Check sheet for the modelled part. Datum: model origin and axes. Units: mm. Give positions to 0.01 mm unless a question says otherwise; leave off trailing zeros. Answer in a Markdown table with one row per item.
from build123d import *

# Parameters (mm, degrees)
EXTRUDE_4_DEPTH = 155


with BuildPart() as part:
    # 草图1 → 凸台-拉伸4 (new body)
    with BuildSketch(Plane.XY):
        with BuildLine():
            Line((1.654438254, 0.021809694), (0.999524111, 15.021809694))
            ThreePointArc((0.999524111, 15.021809694), (0.489092557, 15.499881014), (0, 15))
            Line((0, 15), (0, 0))
            Line((0, 0), (0.5, 0))
            Line((0.5, 0), (0.5, 15))
            Line((0.5, 15), (1.154914144, 0))
            ThreePointArc((1.154914144, 0), (1.654438254, -0.478190306), (2.153962365, 0))
            Line((2.153962365, 0), (2.808876509, 15))
            Line((2.808876509, 15), (3.463790652, 0))
            ThreePointArc((3.463790652, 0), (3.963314763, -0.478190306), (4.462838874, 0))
            Line((4.462838874, 0), (5.117753018, 15))
            Line((5.117753018, 15), (5.772667161, 0))
            ThreePointArc((5.772667161, 0), (6.272191272, -0.478190306), (6.771715383, 0))
            Line((6.771715383, 0), (7.426629527, 15))
            Line((7.426629527, 15), (8.08154367, 0))
            ThreePointArc((8.08154367, 0), (8.581067781, -0.478190306), (9.080591892, 0))
            Line((9.080591892, 0), (9.735506035, 15))
            Line((9.735506035, 15), (10.390420179, 0))
            ThreePointArc((10.390420179, 0), (10.88994429, -0.478190306), (11.389468401, 0))
            Line((11.389468401, 0), (12.044382544, 15))
            Line((12.044382544, 15), (12.699296688, 0))
            ThreePointArc((12.699296688, 0), (13.198820799, -0.478190306), (13.698344909, 0))
            Line((13.698344909, 0), (14.353259053, 15))
            Line((14.353259053, 15), (15.008173197, 0))
            ThreePointArc((15.008173197, 0), (15.507697307, -0.478190306), (16.007221418, 0))
            Line((16.007221418, 0), (16.662135562, 15))
            Line((16.662135562, 15), (17.317049705, 0))
            ThreePointArc((17.317049705, 0), (17.816573816, -0.478190306), (18.316097927, 0))
            Line((18.316097927, 0), (18.971012071, 15))
            Line((18.971012071, 15), (19.625926214, 0))
            ThreePointArc((19.625926214, 0), (20.125450325, -0.478190306), (20.624974436, 0))
            Line((20.624974436, 0), (21.27988858, 15))
            Line((21.27988858, 15), (21.934802723, 0))
            ThreePointArc((21.934802723, 0), (22.434326834, -0.478190306), (22.933850945, 0))
            Line((22.933850945, 0), (23.588765088, 15))
            Line((23.588765088, 15), (24.243679232, 0))
            ThreePointArc((24.243679232, 0), (24.743203343, -0.478190306), (25.242727454, 0))
            Line((25.242727454, 0), (25.897641597, 15))
            Line((25.897641597, 15), (26.552555741, 0))
            ThreePointArc((26.552555741, 0), (27.052079852, -0.478190306), (27.551603962, 0))
            Line((27.551603962, 0), (28.206518106, 15))
            Line((28.206518106, 15), (28.86143225, 0))
            ThreePointArc((28.86143225, 0), (29.36095636, -0.478190306), (29.860480471, 0))
            Line((29.860480471, 0), (30.515394615, 15))
            Line((30.515394615, 15), (31.170308759, 0))
            ThreePointArc((31.170308759, 0), (31.669832869, -0.478190306), (32.16935698, 0))
            Line((32.16935698, 0), (32.824271124, 15))
            Line((32.824271124, 15), (33.479185267, 0))
            ThreePointArc((33.479185267, 0), (33.978709378, -0.478190306), (34.478233489, 0))
            Line((34.478233489, 0), (35.133147633, 15))
            Line((35.133147633, 15), (35.788061776, 0))
            ThreePointArc((35.788061776, 0), (36.287585887, -0.478190306), (36.787109998, 0))
            Line((36.787109998, 0), (37.442024141, 15))
            Line((37.442024141, 15), (37.442024141, 0))
            Line((37.442024141, 0), (37.942024141, 0))
            Line((37.942024141, 0), (37.942024141, 15))
            ThreePointArc((37.942024141, 15), (37.452931584, 15.499881014), (36.942500031, 15.021809694))
            Line((36.942500031, 15.021809694), (36.287585887, 0.021809694))
            Line((36.287585887, 0.021809694), (35.632671743, 15.021809694))
            ThreePointArc((35.632671743, 15.021809694), (35.133147633, 15.5), (34.633623522, 15.021809694))
            Line((34.633623522, 15.021809694), (33.978709378, 0.021809694))
            Line((33.978709378, 0.021809694), (33.323795235, 15.021809694))
            ThreePointArc((33.323795235, 15.021809694), (32.824271124, 15.5), (32.324747013, 15.021809694))
            Line((32.324747013, 15.021809694), (31.669832869, 0.021809694))
            Line((31.669832869, 0.021809694), (31.014918726, 15.021809694))
            ThreePointArc((31.014918726, 15.021809694), (30.515394615, 15.5), (30.015870504, 15.021809694))
            Line((30.015870504, 15.021809694), (29.36095636, 0.021809694))
            Line((29.36095636, 0.021809694), (28.706042217, 15.021809694))
            ThreePointArc((28.706042217, 15.021809694), (28.206518106, 15.5), (27.706993995, 15.021809694))
            Line((27.706993995, 15.021809694), (27.052079852, 0.021809694))
            Line((27.052079852, 0.021809694), (26.397165708, 15.021809694))
            ThreePointArc((26.397165708, 15.021809694), (25.897641597, 15.5), (25.398117486, 15.021809694))
            Line((25.398117486, 15.021809694), (24.743203343, 0.021809694))
            Line((24.743203343, 0.021809694), (24.088289199, 15.021809694))
            ThreePointArc((24.088289199, 15.021809694), (23.588765088, 15.5), (23.089240978, 15.021809694))
            Line((23.089240978, 15.021809694), (22.434326834, 0.021809694))
            Line((22.434326834, 0.021809694), (21.77941269, 15.021809694))
            ThreePointArc((21.77941269, 15.021809694), (21.27988858, 15.5), (20.780364469, 15.021809694))
            Line((20.780364469, 15.021809694), (20.125450325, 0.021809694))
            Line((20.125450325, 0.021809694), (19.470536181, 15.021809694))
            ThreePointArc((19.470536181, 15.021809694), (18.971012071, 15.5), (18.47148796, 15.021809694))
            Line((18.47148796, 15.021809694), (17.816573816, 0.021809694))
            Line((17.816573816, 0.021809694), (17.161659673, 15.021809694))
            ThreePointArc((17.161659673, 15.021809694), (16.662135562, 15.5), (16.162611451, 15.021809694))
            Line((16.162611451, 15.021809694), (15.507697307, 0.021809694))
            Line((15.507697307, 0.021809694), (14.852783164, 15.021809694))
            ThreePointArc((14.852783164, 15.021809694), (14.353259053, 15.5), (13.853734942, 15.021809694))
            Line((13.853734942, 15.021809694), (13.198820799, 0.021809694))
            Line((13.198820799, 0.021809694), (12.543906655, 15.021809694))
            ThreePointArc((12.543906655, 15.021809694), (12.044382544, 15.5), (11.544858433, 15.021809694))
            Line((11.544858433, 15.021809694), (10.88994429, 0.021809694))
            Line((10.88994429, 0.021809694), (10.235030146, 15.021809694))
            ThreePointArc((10.235030146, 15.021809694), (9.735506035, 15.5), (9.235981925, 15.021809694))
            Line((9.235981925, 15.021809694), (8.581067781, 0.021809694))
            Line((8.581067781, 0.021809694), (7.926153637, 15.021809694))
            ThreePointArc((7.926153637, 15.021809694), (7.426629527, 15.5), (6.927105416, 15.021809694))
            Line((6.927105416, 15.021809694), (6.272191272, 0.021809694))
            Line((6.272191272, 0.021809694), (5.617277128, 15.021809694))
            ThreePointArc((5.617277128, 15.021809694), (5.117753018, 15.5), (4.618228907, 15.021809694))
            Line((4.618228907, 15.021809694), (3.963314763, 0.021809694))
            Line((3.963314763, 0.021809694), (3.30840062, 15.021809694))
            ThreePointArc((3.30840062, 15.021809694), (2.808876509, 15.5), (2.309352398, 15.021809694))
            Line((2.309352398, 15.021809694), (1.654438254, 0.021809694))
        make_face()
    extrude(amount=EXTRUDE_4_DEPTH)


solid = part.part
(1) Mould release check, pull along X, two halves, no side actions. Record for faces 1 (the flat face through (23, 8, 155)), 2 (the flat face through (1.33, 7.42, 76.41)): pulls with the +X half, pulls with the -X half, needs draft (parallel to the pull), parting line crosses it, or undercut.
Geometry says:
| item | result |
|---|---|
| face 1 | needs draft |
| face 2 | undercut |
(2) Gauge pin test, flat end, axial feed: P1, Ø0.6, axis at x = 0, z = 66.5, coming from the -Y side. Record the tip position at first contact, or that the pin passes through.
Geometry says:
| item | result |
|---|---|
| P1 | y = 0 |
(3) Cross-section at A-A, the plane y = 5. Give the number of separate pieces and of enclosed holes in the cut face, then the cut area to 3 significant figures.
Geometry says:
| item | result |
|---|---|
| separate pieces | 34 |
| enclosed holes | 0 |
| area | 2,640 mm² |
